Check sheet for the modelled part. Datum: model origin and axes. Units: mm. Face numbers are marked on the shaded views. A direction names the side the tool comes from. Round coordinates to 2 decimals unless told otherwise and drop trailing zeros. Write each loop counter-clockwise with the first axis right and the second up, starting at its lowest first coordinate (ties: lowest second). Pieces come first, ordered by that corner, then holes.
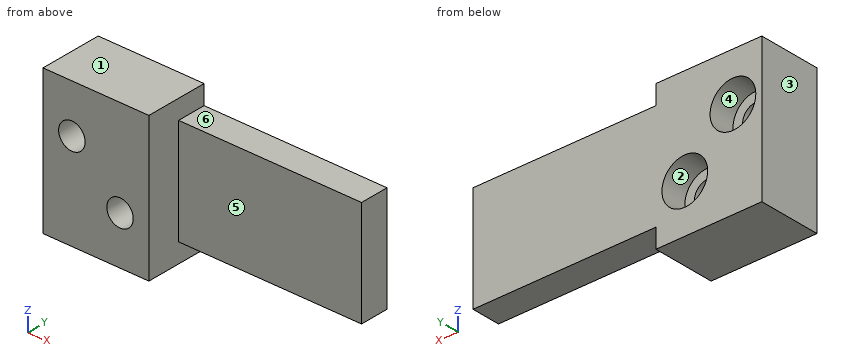
from build123d import *

# Parameters (mm, degrees)
ESBO_O1_W                  = 38
ESBO_O1_H                  = 6
RESSALTO_EXTRUS_O1_DEPTH   = 30
CORTE_EXTRUS_O1_DEPTH      = 69.330081223
CORTE_EXTRUS_O1_DEPTH_BACK = 69.330081223
ESBO_O2_W                  = 38
ESBO_O2_H                  = 4
CORTE_EXTRUS_O2_DEPTH      = 69.330081223
CORTE_EXTRUS_O2_DEPTH_BACK = 69.330081223
ESBO_O4_R                  = 2.75
ESBO_O5_R                  = 4.75
CORTE_EXTRUS_O3_DEPTH      = 5.4


with BuildPart() as part:
    # Esboço1 → Ressalto-extrusão1 (new body)
    with BuildSketch(Plane.XY):
        Polygon((22, 0), (0, 0), (0, -13), (22, -13), (22, -6), align=None)
        with Locations((41, -3)):
            Rectangle(ESBO_O1_W, ESBO_O1_H)
    extrude(amount=RESSALTO_EXTRUS_O1_DEPTH)

    # Esboço2 → Corte-extrusão1 (cut, two sides: drawn at the far end of the back side and taken through both)
    with BuildSketch(Plane(origin=(0, 0, 0), x_dir=(1, 0, 0), z_dir=(0, 1, 0)).offset(-CORTE_EXTRUS_O1_DEPTH_BACK)):
        with Locations((41, -2)):
            Rectangle(ESBO_O2_W, ESBO_O2_H)
        with Locations((41, -28)):
            Rectangle(ESBO_O2_W, ESBO_O2_H)
    extrude(amount=CORTE_EXTRUS_O1_DEPTH + CORTE_EXTRUS_O1_DEPTH_BACK, mode=Mode.SUBTRACT)

    # Esboço4 → Corte-extrusão2 (cut, two sides: drawn at the far end of the back side and taken through both)
    with BuildSketch(Plane(origin=(0, 0, 0), x_dir=(1, 0, 0), z_dir=(0, 1, 0)).offset(-CORTE_EXTRUS_O2_DEPTH_BACK)):
        with Locations(Location((6, -20, 0), (0, 0, 270))):
            Circle(ESBO_O4_R)
        with Locations(Location((16, -10, 0), (0, 0, 270))):
            Circle(ESBO_O4_R)
    extrude(amount=CORTE_EXTRUS_O2_DEPTH + CORTE_EXTRUS_O2_DEPTH_BACK, mode=Mode.SUBTRACT)

    # Esboço5 → Corte-extrusão3 (cut)
    with BuildSketch(Plane(origin=(0, 0, 0), x_dir=(1, 0, 0), z_dir=(0, 1, 0))):
        with Locations(Location((6, -20, 0), (0, 0, 270))):
            Circle(ESBO_O5_R)
        with Locations(Location((16, -10, 0), (0, 0, 270))):
            Circle(ESBO_O5_R)
    extrude(amount=-CORTE_EXTRUS_O3_DEPTH, mode=Mode.SUBTRACT)


solid = part.part
1. Sectioned sample at D-D, the plane z = 23.5. Enter the section's corners in (x, y).
2. Sectioned sample at A-A, the plane z = 20. Enter the section's corners in (x, y), plus the area to 3 significant figures.
3. Sectioned sample at C-C, the plane y = -4. Enter the section's corners in (x, z).
4. Set-up check for the marked faces 4, 5 and 6: record each of +Z, -Z, +X, -X, +Y, -Y from which the full face is reachable in a straight line by a thin tool's end or side.
5. Release check for a two-part mould opening along X. For the marked faces 1, 2 and 3 record: released by +X, released by -X, zero draft, split by the parting line, or undercut.
6. Go/stop test with flat-tipped pins: pin 1 (3 mm diameter, centred on x = 38, y = -2, fed in from +Z); pin 2 (5 mm diameter, centred on x = 6, z = 20, fed in from -Y); pin 3 (5 mm diameter, centred on x = 16.5, z = 11, fed in from +Y); pin 4 (6.5 mm diameter, centred on x = 40.5, y = -1.5, fed in from -Z). Record where each tip stops, or that it passes through.
7. Scan lines: line 1 along Z through (x, y) = (16, -7.5); line 2 along X through (y, z) = (-1.3, 10); line 3 along Y through (x, z) = (41, 9.25). Record each from-to range of solid material in increasing order.
8. Sectioned sample at B-B, the plane x = 6. Enter the section's corners in (y, z), plus the area to 3 significant figures.
Computed values:
1. outline: (0, -13) - (22, -13) - (22, -6) - (60, -6) - (60, 0) - (9.21, 0) - (9.21, -5.4) - (2.79, -5.4) - (2.79, 0) - (0, 0) - close
2. outline: (0, -13) - (3.25, -13) - (3.25, -5.4) - (1.25, -5.4) - (1.25, 0) - (0, 0) - close; (8.75, -13) - (22, -13) - (22, -6) - (60, -6) - (60, 0) - (10.75, 0) - (10.75, -5.4) - (8.75, -5.4) - close
2. area: 421 mm2
3. outline: (0, 0) - (22, 0) - (22, 4) - (60, 4) - (60, 26) - (22, 26) - (22, 30) - (0, 30) - close; hole circle Ø9.5 at (6, 20); hole circle Ø9.5 at (16, 10)
4. face 4: +Y
4. face 5: +Z, -Z, +X, -Y
4. face 6: +Z, +X, +Y, -Y
5. face 1: zero draft
5. face 2: undercut
5. face 3: released by -X
6. pin 1: stops at z = 26
6. pin 2: passes through
6. pin 3: stops at y = -5.4
6. pin 4: stops at z = 4
7. line 1: z = 0 to 7.25, 12.75 to 30
7. line 2: x = 0 to 11.25, 20.75 to 60
7. line 3: y = -6 to 0
8. outline: (-13, 0) - (0, 0) - (0, 15.25) - (-5.4, 15.25) - (-5.4, 17.25) - (-13, 17.25) - close; (-13, 22.75) - (-5.4, 22.75) - (-5.4, 24.75) - (0, 24.75) - (0, 30) - (-13, 30) - close
8. area: 297 mm2
